The model under review builds one solid part; all positions refer to its coordinate system, in mm. Face numbers are marked on the shaded views. A direction names the side the tool comes from. Round coordinates to 2 decimals unless told otherwise and drop trailing zeros. Order: outer loops, then holes, each group sorted by start corner. A loop starts at its lowest first (then second) coordinate and runs counter-clockwise, first axis right, second up. Notation, with made-up numbers: (4, -23) -> (47, -23) arc R23 ccw to (47, 14) -> close; hole circle Ø7 at (70.25, 60.5). An arc over 180 degrees is marked (long way). Use a Markdown table: item, result. Add a question column.
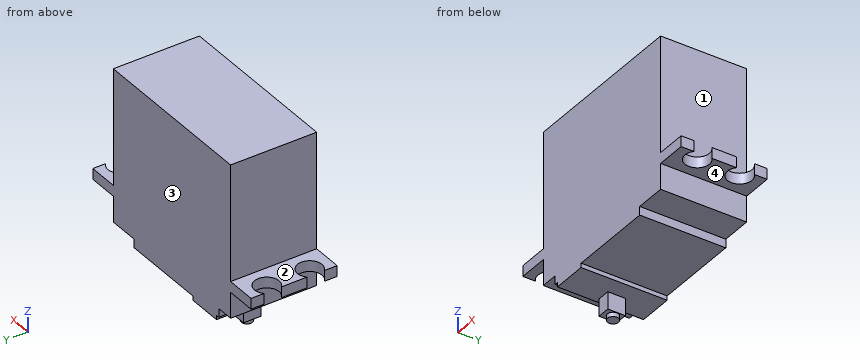
```python
from build123d import *

# Parameters (mm, degrees)
BOSS_EXTRUDE1_DEPTH     = 20
SKETCH2_W               = 3.154933035
SKETCH2_H               = 9.663476497
CUT_EXTRUDE1_DEPTH      = 4
SKETCH3_W               = 3
SKETCH3_H               = 7
CUT_EXTRUDE2_DEPTH      = 4
SKETCH4_R               = 1.281422033
BOSS_EXTRUDE3_DEPTH     = 1
CUT_EXTRUDE3_DEPTH      = 79.790553635
CUT_EXTRUDE3_DEPTH_BACK = 79.790553635
CUT_EXTRUDE4_DEPTH      = 79.790553635
CUT_EXTRUDE4_DEPTH_BACK = 79.790553635


with BuildPart() as part:
    # Sketch1 → Boss-Extrude1 (new body)
    with BuildSketch(Plane(origin=(0, 0, 0), x_dir=(1, 0, 0), z_dir=(0, 1, 0))):
        Polygon((-59.245647318, 22.93293572), (-63.268779285, 22.93293572), (-63.268779285, 16.93293572), (-70.268779285, 16.93293572), (-70.268779285, 14.43293572), (-63.268779285, 14.43293572), (-63.268779285, -12.56706428), (-23.268779285, -12.56706428), (-23.268779285, 14.43293572), (-16.268779285, 14.43293572), (-16.268779285, 16.93293572), (-23.268779285, 16.93293572), (-23.268779285, 22.93293572), (-30.393090753, 22.93293572), (-30.393090753, 24.93293572), (-50.386032487, 24.93293572), (-50.386032487, 25.935013561), (-54.386032487, 25.935013561), (-54.386032487, 29.935013561), (-57.386032487, 29.935013561), (-57.386032487, 25.935013561), (-58.4541935, 25.935013561), (-58.4541935, 24.93293572), (-59.245647318, 24.93293572), align=None)
    extrude(amount=BOSS_EXTRUDE1_DEPTH)

    # Sketch2 → Cut-Extrude1 (cut)
    with BuildSketch(Plane(origin=(0, 0, -25.935013561), x_dir=(-1, 0, 0), z_dir=(0, 0, -1))):
        with Locations((55.851514708, 4.096059823)):
            Rectangle(SKETCH2_W, SKETCH2_H)
    extrude(amount=CUT_EXTRUDE1_DEPTH, mode=Mode.SUBTRACT)

    # Sketch3 → Cut-Extrude2 (cut)
    with BuildSketch(Plane(origin=(0, 0, -29.935013561), x_dir=(-1, 0, 0), z_dir=(0, 0, -1))):
        with Locations((55.886032487, 16.5)):
            Rectangle(SKETCH3_W, SKETCH3_H)
    extrude(amount=-CUT_EXTRUDE2_DEPTH, mode=Mode.SUBTRACT)

    # Sketch4 → Boss-Extrude3 (add)
    with BuildSketch(Plane(origin=(0, 0, -29.935013561), x_dir=(-1, 0, 0), z_dir=(0, 0, -1))):
        with Locations(Location((55.79519526, 11.102128328, 0), (0, 0, 180))):
            Circle(SKETCH4_R)
    extrude(amount=BOSS_EXTRUDE3_DEPTH)

    # Sketch5 → Cut-Extrude3 (cut, two sides: drawn at the far end of the back side and taken through both)
    with BuildSketch(Plane(origin=(0, 0, -16.93293572), x_dir=(-1, 0, 0), z_dir=(0, 0, -1)).offset(-CUT_EXTRUDE3_DEPTH_BACK)):
        with BuildLine():
            Line((70.268779285, 12.977163389), (70.268779285, 17))
            ThreePointArc((70.268779285, 17), (65.412785932, 14.988581694), (70.268779285, 12.977163389))
        make_face()
        with BuildLine():
            Line((70.268779285, 3), (70.268779285, 7.004039222))
            ThreePointArc((70.268779285, 7.004039222), (65.403430944, 5.002019611), (70.268779285, 3))
        make_face()
    extrude(amount=CUT_EXTRUDE3_DEPTH + CUT_EXTRUDE3_DEPTH_BACK, mode=Mode.SUBTRACT)

    # Sketch6 → Cut-Extrude4 (cut, two sides: drawn at the far end of the back side and taken through both)
    with BuildSketch(Plane(origin=(0, 0, -16.93293572), x_dir=(-1, 0, 0), z_dir=(0, 0, -1)).offset(-CUT_EXTRUDE4_DEPTH_BACK)):
        with BuildLine():
            Line((16.268779285, 17), (16.268779285, 12.89909256))
            ThreePointArc((16.268779285, 12.89909256), (21.084964529, 14.94954628), (16.268779285, 17))
        make_face()
        with BuildLine():
            Line((16.268779285, 7.134169091), (16.268779285, 3))
            ThreePointArc((16.268779285, 3), (21.067521343, 5.067084545), (16.268779285, 7.134169091))
        make_face()
    extrude(amount=CUT_EXTRUDE4_DEPTH + CUT_EXTRUDE4_DEPTH_BACK, mode=Mode.SUBTRACT)


solid = part.part
```
Q1. Add section D-D (y = 6.25). Write out the cut boundary in (x, z), then the cut area to 3 significant figures.
Q2. Add section A-A (y = 18.5). Write out the cut boundary in (x, z).
Q3. Add section C-C (z = -18). Write out the cut boundary in (x, y).
Q4. Machinability: for the marked faces 1, 2, 3 and 4, which of the approach directions +Z, -Z, +X, -X, +Y, -Y give a long, thin tool a straight path to every point of the face, cutting with its end or side? Answer none if there is none.
Q5. Add section B-B (x = -26.5). Write out the cut boundary in (y, z), then the cut area to 3 significant figures.
Q6. Wall thickness on line 1 (Z direction, x = -27.5, y = 4.5); line 2 (X direction, y = 11, z = -7.5); line 3 (Z direction, x = -58, y = 7): over which ranges is each line inside the solid? List them lowest first. Write a range as [from, to].
Q7. Insertion check: pin 1 (2 mm diameter, centred on y = 11, z = -27.5, fed in from +X); pin 2 (3 mm diameter, centred on y = 13, z = -12.5, fed in from +X); pin 3 (6 mm diameter, centred on x = -41.5, z = -18.5, fed in from -Y); pin 4 (3.5 mm diameter, centred on x = -18.24, y = 14.95, fed in from -Z). Each pin has a flat end and moves straight along its axis. Give the tip position at first contact, or say it passes through.
Report:
| question | item | result |
|---|---|---|
| 1 | outline | (-65.69, -16.93) -> (-63.27, -16.93) -> (-63.27, -22.93) -> (-59.25, -22.93) -> (-59.25, -24.93) -> (-58.45, -24.93) -> (-58.45, -25.94) -> (-50.39, -25.94) -> (-50.39, -24.93) -> (-30.39, -24.93) -> (-30.39, -22.93) -> (-23.27, -22.93) -> (-23.27, -16.93) -> (-20.81, -16.93) -> (-20.81, -14.43) -> (-23.27, -14.43) -> (-23.27, 12.57) -> (-63.27, 12.57) -> (-63.27, -14.43) -> (-65.69, -14.43) -> close |
| 1 | area | 1,500 mm² |
| 2 | outline | (-70.27, -16.93) -> (-63.27, -16.93) -> (-63.27, -22.93) -> (-59.25, -22.93) -> (-59.25, -24.93) -> (-58.45, -24.93) -> (-58.45, -25.94) -> (-50.39, -25.94) -> (-50.39, -24.93) -> (-30.39, -24.93) -> (-30.39, -22.93) -> (-23.27, -22.93) -> (-23.27, -16.93) -> (-16.27, -16.93) -> (-16.27, -14.43) -> (-23.27, -14.43) -> (-23.27, 12.57) -> (-63.27, 12.57) -> (-63.27, -14.43) -> (-70.27, -14.43) -> close |
| 3 | outline | (-63.27, 0) -> (-23.27, 0) -> (-23.27, 20) -> (-63.27, 20) -> close |
| 4 | face 1 | +Z, +X, +Y, -Y |
| 4 | face 2 | +Z, -X, +Y, -Y |
| 4 | face 3 | +Z, -Z, +X, -X, +Y |
| 4 | face 4 | -Z, +X, +Y, -Y |
| 5 | outline | (0, -22.93) -> (20, -22.93) -> (20, 12.57) -> (0, 12.57) -> close |
| 5 | area | 710 mm² |
| 6 | line 1 | z = [-22.93, 12.57] |
| 6 | line 2 | x = [-63.27, -23.27] |
| 6 | line 3 | z = [-25.94, 12.57] |
| 7 | pin 1 | stops at x = -54.39 |
| 7 | pin 2 | stops at x = -23.27 |
| 7 | pin 3 | stops at y = 0 |
| 7 | pin 4 | passes through |
